Read the model definition and answer for the solid it produces. Units are mm, in the model's axes. Face numbers are marked on the shaded views. A direction names the side the tool comes from. Round coordinates to 2 decimals unless told otherwise and drop trailing zeros. Write each loop counter-clockwise with the first axis right and the second up, starting at its lowest first coordinate (ties: lowest second). Pieces come first, ordered by that corner, then holes. Notation, with made-up numbers: (52.5, -14) - (97.5, -14) arc R6 ccw to (97.5, -5) - close; hole circle Ø6 at (18, 88.25). An arc over 180 degrees is marked (long way). One line per item, written item: value. Start each with the question number.
(1) Find the intervals of material crossed by L1, parallel to Y at x = -10, z = -2; L2, parallel to X at y = 0.5, z = 8; L3, parallel to X at y = 4, z = 2.75, in increasing order.
(2) A cutting plane is placed at C-C, the plane x = -6.75. Determine the outline of the cut face in (y, z), plus the area to 3 significant figures.
(3) A cutting plane is placed at B-B, the plane y = -0.75. Determine the outline of the cut face in (x, z), plus the area to 3 significant figures.
(4) Flat-ended cylindrical pins translate along their axes: pin 1 Ø2 at (x, y) = (-6, 3) entering from +Z; pin 2 Ø1 at (y, z) = (3.5, 2.5) entering from -X; pin 3 Ø5 at (x, z) = (-8, -5) entering from +Y. Find the tip coordinate at first contact, or state that the pin passes through.
(5) For the marked faces 1 and 2, determine the directions among +Z, -Z, +X, -X, +Y, -Y from which every point of the face is accessible in a straight line to the end or side of a thin tool.
(6) A cutting plane is placed at D-D, the plane y = 4.5. Determine the outline of the cut face in (x, z).
(7) A cutting plane is placed at A-A, the plane z = 0. Determine the outline of the cut face in (x, y).
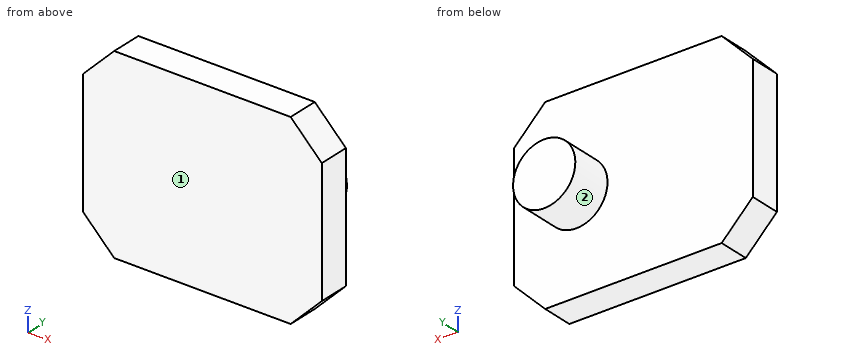
from build123d import *

# Parameters (mm, degrees)
SKETCH_1_W      = 23
SKETCH_1_H      = 18
EXTRUDE_1_DEPTH = 1.5
CHAMFER_1_SIZE  = 3
SKETCH_2_R      = 3
EXTRUDE_2_DEPTH = 4


with BuildPart() as part:
    # 草图1 → 凸台-拉伸1 (new, symmetric)
    with BuildSketch(Plane(origin=(0, 0, 0), x_dir=(1, 0, 0), z_dir=(0, 1, 0))):
        Rectangle(SKETCH_1_W, SKETCH_1_H)
    extrude(amount=EXTRUDE_1_DEPTH, both=True)

    # 倒角1
    chamfer_1_edges = [part.edges().sort_by_distance(p)[0] for p in [
        (11.5, 0, 9),
        (-11.5, 0, 9),
        (-11.5, 0, -9),
        (11.5, 0, -9),
    ]]
    chamfer(chamfer_1_edges, length=CHAMFER_1_SIZE)

    # 草图2 → 凸台-拉伸2 (add)
    with BuildSketch(Plane(origin=(0, 1.5, 0), x_dir=(1, 0, 0), z_dir=(0, 1, 0))):
        with Locations(Location((5.5, 0, 0), (0, 0, 270))):
            Circle(SKETCH_2_R)
    extrude(amount=EXTRUDE_2_DEPTH)


solid = part.part
Here are the results:
1. L1: -1.5 to 1.5
1. L2: -9.5 to 9.5
1. L3: 4.3 to 6.7
2. outline: (-1.5, -9) - (1.5, -9) - (1.5, 9) - (-1.5, 9) - close
2. area: 54.0 mm²
3. outline: (-11.5, -6) - (-8.5, -9) - (8.5, -9) - (11.5, -6) - (11.5, 6) - (8.5, 9) - (-8.5, 9) - (-11.5, 6) - close
3. area: 396 mm²
4. pin 1: through
4. pin 2: x = 3.26
4. pin 3: y = 1.5
5. face 1: +Z, -Z, +X, -X, -Y
5. face 2: +Y
6. outline: circle Ø6 at (5.5, 0)
7. outline: (-11.5, -1.5) - (11.5, -1.5) - (11.5, 1.5) - (8.5, 1.5) - (8.5, 5.5) - (2.5, 5.5) - (2.5, 1.5) - (-11.5, 1.5) - close
